Geometry: see drawing. Coordinates: mm, zero at the bounding-box minimum. Give positions to 0.01 mm unless a question says otherwise; leave off trailing zeros. Write each loop counter-clockwise with the first axis right and the second up, starting at its lowest first coordinate (ties: lowest second). Pieces come first, ordered by that corner, then holes. Notation, with made-up numbers: (-10.5, 47) -> (3.5, 47) arc R11 cw to (3.5, 57) -> close; hole circle Ø1 at (84.5, 11). An arc over 180 degrees is marked (long way). Write item = value, one per line.
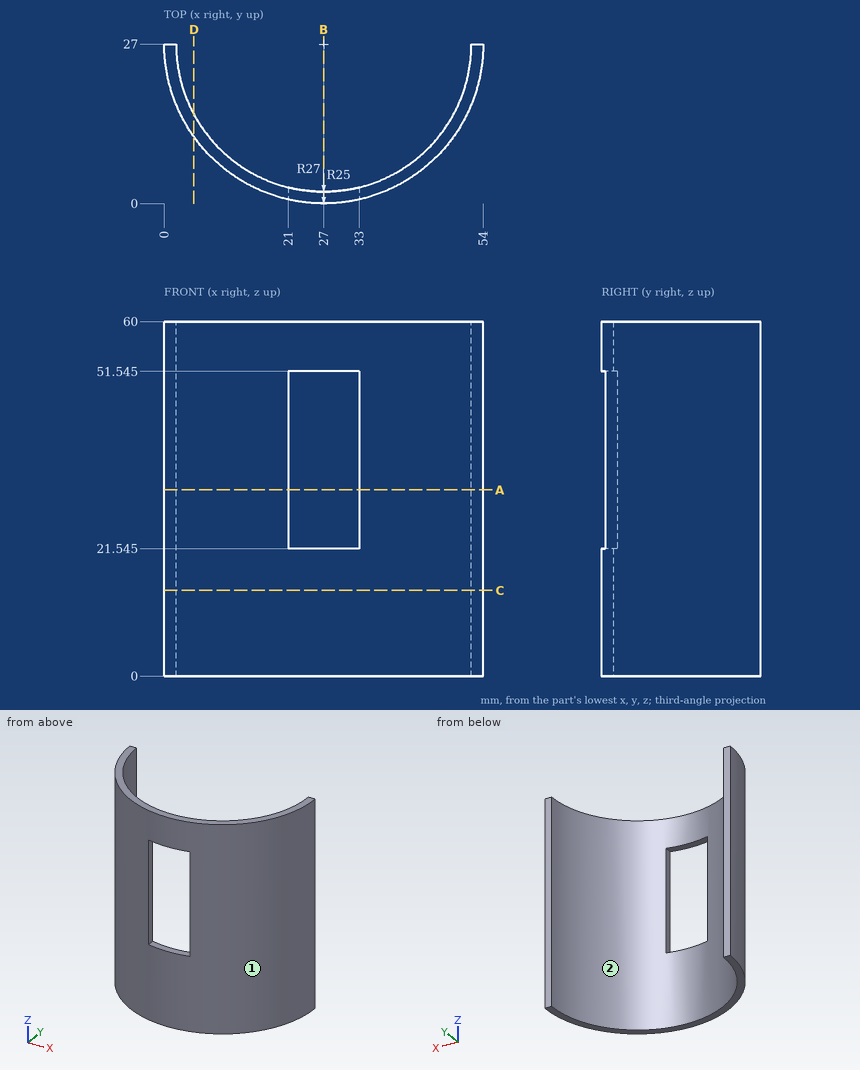
(1) Section query A-A (z = 31.5). Return loops of the section in (x, y).
Values follow:
outline = (0, 27) arc R27 ccw to (21, 0.68) -> (21, 2.73) arc R25 cw to (2, 27) -> close; (33, 0.68) arc R27 ccw to (54, 27) -> (52, 27) arc R25 cw to (33, 2.73) -> close
(2) Material intervals for line 1 (X direction, y = 14, z = 22.5); line 2 (X direction, y = 7.5, z = 42) (1 decimal); line 3 (Y direction, x = 28, z = 15.5), sorted ascending.
Values follow:
line_1 = 3.34 to 5.65, 48.35 to 50.66
line_2 = 8.3 to 11.4, 42.6 to 45.7
line_3 = 0.02 to 2.02
(3) Section query D-D (x = 5). Return loops of the section in (y, z).
Values follow:
outline = (11.35, 0) -> (15.13, 0) -> (15.13, 60) -> (11.35, 60) -> close
(4) Section query C-C (z = 14.5). Return loops of the section in (x, y).
Values follow:
outline = (0, 27) arc R27 ccw to (54, 27) -> (52, 27) arc R25 cw to (2, 27) -> close
(5) Pull-direction query (X, two-part tool) for the marked faces 1 and 2; classes: pulls with the +X half, pulls with the -X half, needs draft (parallel to the pull), parting line crosses it, or undercut.
Values follow:
face_1 = parting line crosses it
face_2 = undercut
(6) First-contact query: pin 1 (12 mm diameter, centred on y = 10, z = 35.5, fed in from -X); pin 2 (1 mm diameter, centred on y = 2, z = 41, fed in from -X); pin 3 (6 mm diameter, centred on y = 14, z = 21.5, fed in from +X). Flat tips, straight axial feed; report the tip coordinate or a pass-through.
Values follow:
pin_1 = 2.34
pin_2 = 15.65
pin_3 = 52.08
(7) Section query B-B (x = 27). Return loops of the section in (y, z) (3 decimals).
Values follow:
outline = (0, 0) -> (2, 0) -> (2, 21.545) -> (0, 21.545) -> close; (0, 51.545) -> (2, 51.545) -> (2, 60) -> (0, 60) -> close
